Build history of the part. All positions in model axes, mm. A direction names the side the tool comes from. Give positions to 0.01 mm unless a question says otherwise; leave off trailing zeros. Order: outer loops, then holes, each group sorted by start corner. A loop starts at its lowest first (then second) coordinate and runs counter-clockwise, first axis right, second up. Notation, with made-up numbers: (87, 29) - (101, 29) arc R9 cw to (101, 42) - close; hole circle Ø2 at (-27.75, -15.75). An arc over 180 degrees is marked (long way). Use a Markdown table: item, result. Add a question column.
(1) Slice it at A-A (z = -39). Write the cut outline in (x, y).
(2) Flat gauge pins, fed straight in: pin 1 (6 mm diameter, centred on x = 223, y = 4.5, fed in from +Z); pin 2 (11.5 mm diameter, centred on x = 39.03, z = -19.51, fed in from -Y); pin 3 (6 mm diameter, centred on x = 59, y = 79, fed in from +Z). Where does each tip first touch, or does it go through?
(3) Which spindle directions (+Z, -Z, +X, -X, +Y, -Y) get a long thin tool onto all of the face, cutting with end or side? Do faces 4 (the face through (155, 7.62, -69)), 5 (the face through (138.825, 97.843, -52.046)), 6 (the face through (221.732, 95.161, -148.505)). Say none if no direction does.
(4) Slice it at D-D (y = 43). Write the cut outline in (x, z).
(5) Wall check: line 1 (Y direction, x = 155.5, z = -60.5); line 2 (X direction, y = 6.5, z = -4); line 3 (X direction, y = 96.5, z = 0). Give the ranges that are in metal, low to high.
(6) Slice it at B-B (x = 162). Write the cut outline in (y, z), then the cut area to 3 significant figures.
(7) Mould opens along X. For faces 1 (the face through (89, 95, -89)), 2 (the face through (143, 93.98, -52)), 3 (the face through (194.36, 6.26, -166.13)) say: +X half, -X half, draft (parallel to the pull), parting line (faces both ways), or undercut.
(8) Slice it at C-C (z = -3). Write the cut outline in (x, y).
from build123d import *

# Parameters (mm, degrees)
BOSS_EXTRUDE1_DEPTH = 101.6
SKETCH2_W           = 267.926874414
SKETCH2_H           = 76.2
CUT_EXTRUDE1_DEPTH  = 71.12
SKETCH3_R           = 6.35
CUT_EXTRUDE3_DEPTH  = 313.194791695
CUT_EXTRUDE4_DEPTH  = 7.62
CUT_EXTRUDE5_DEPTH  = 7.62


with BuildPart() as part:
    # Sketch1 → Boss-Extrude1 (new body)
    with BuildSketch(Plane(origin=(0, 0, 0), x_dir=(1, 0, 0), z_dir=(0, 1, 0))):
        Polygon((0, 0), (179.605122421, 179.605122421), (209.535625582, 152.272255569), (234.275538547, 144.630280974), (62.844388347, -43.093188015), align=None)
    extrude(amount=BOSS_EXTRUDE1_DEPTH)

    # Sketch2 → Cut-Extrude1 (cut)
    with BuildSketch(Plane(origin=(0, 0, 0), x_dir=(-0.7071067811865464, 0, 0.7071067811865487), z_dir=(-0.7071067811865487, 0, -0.7071067811865464))):
        with Locations((-133.963437207, 50.8)):
            Rectangle(SKETCH2_W, SKETCH2_H)
    extrude(amount=-CUT_EXTRUDE1_DEPTH, mode=Mode.SUBTRACT)

    # Sketch3 → Cut-Extrude3 (cut, through all)
    with BuildSketch(Plane(origin=(0, 101.6, 0), x_dir=(1, 0, 0), z_dir=(0, 1, 0))):
        with Locations(Location((21.07252481, 1.552947287, 0), (0, 0, 270))):
            Circle(SKETCH3_R)
        with Locations(Location((39.033037052, 19.513459529, 0), (0, 0, 270))):
            Circle(SKETCH3_R)
        with Locations(Location((56.993549294, 37.473971772, 0), (0, 0, 270))):
            Circle(SKETCH3_R)
        with Locations(Location((74.954061536, 55.434484014, 0), (0, 0, 270))):
            Circle(SKETCH3_R)
        with Locations(Location((92.914573778, 73.394996256, 0), (0, 0, 270))):
            Circle(SKETCH3_R)
        with Locations(Location((110.87508602, 91.355508498, 0), (0, 0, 270))):
            Circle(SKETCH3_R)
        with Locations(Location((128.835598263, 109.31602074, 0), (0, 0, 270))):
            Circle(SKETCH3_R)
        with Locations(Location((146.796110505, 127.276532982, 0), (0, 0, 270))):
            Circle(SKETCH3_R)
        with Locations(Location((164.756622747, 145.237045224, 0), (0, 0, 270))):
            Circle(SKETCH3_R)
    extrude(amount=-CUT_EXTRUDE3_DEPTH, mode=Mode.SUBTRACT)

    # Sketch4 → Cut-Extrude4 (cut)
    with BuildSketch(Plane(origin=(0, 101.6, 0), x_dir=(1, 0, 0), z_dir=(0, 1, 0))):
        Polygon((57.221000047, -36.701269589), (222.746181499, 143.313374464), (227.72700376, 141.940671831), (60.924166757, -39.463469017), align=None)
    extrude(amount=-CUT_EXTRUDE4_DEPTH, mode=Mode.SUBTRACT)

    # Sketch5 → Cut-Extrude5 (cut)
    with BuildSketch(Plane(origin=(0, 0, 0), x_dir=(-1, 0, 0), z_dir=(0, -1, 0))):
        Polygon((-218.913299563, 144.742548401), (-62.856752097, -25.376237408), (-58.071451081, -30.592741372), (-62.856752097, -34.982483231), (-227.725480711, 144.742548401), align=None)
    extrude(amount=-CUT_EXTRUDE5_DEPTH, mode=Mode.SUBTRACT)


solid = part.part
Solution:
| question | item | result |
|---|---|---|
| 1 | outline | (39, 0) - (50.83, 0) - (50.83, 12.7) - (39, 12.7) - close; (39, 88.9) - (50.83, 88.9) - (50.83, 101.6) - (39, 101.6) - close; (63.16, 0) - (121.91, 0) - (121.91, 7.62) - (130.72, 7.62) - (130.72, 0) - (137.81, 0) - (137.81, 12.7) - (63.16, 12.7) - close; (63.16, 88.9) - (137.81, 88.9) - (137.81, 101.6) - (133.07, 101.6) - (133.07, 93.98) - (126.83, 93.98) - (126.83, 101.6) - (63.16, 101.6) - close |
| 2 | pin 1 | z = -129 |
| 2 | pin 2 | through |
| 2 | pin 3 | z = 42.51 |
| 3 | face 4 | -Y |
| 3 | face 5 | +Y |
| 3 | face 6 | -Z, +X, +Y, -Y |
| 4 | outline | (59.67, 40.91) - (119.23, -18.65) - (62.84, 43.09) - close |
| 5 | line 1 | 0 to 12.7, 88.9 to 101.6 |
| 5 | line 2 | 4 to 15.21, 26.93 to 89.8, 98.62 to 105.85 |
| 5 | line 3 | 0 to 14.92, 27.23 to 90.97, 97.21 to 102.2 |
| 6 | outline | (0, -162) - (12.7, -162) - (12.7, -150.96) - (0, -150.96) - close; (0, -139.52) - (12.7, -139.52) - (12.7, -65.49) - (0, -65.49) - (0, -73.09) - (7.62, -73.09) - (7.62, -82.7) - (0, -82.7) - close; (88.9, -162) - (101.6, -162) - (101.6, -150.96) - (88.9, -150.96) - close; (88.9, -139.52) - (101.6, -139.52) - (101.6, -77.25) - (93.98, -77.25) - (93.98, -70.46) - (101.6, -70.46) - (101.6, -65.49) - (88.9, -65.49) - close |
| 6 | area | 2,040 mm2 |
| 7 | face 1 | -X half |
| 7 | face 2 | undercut |
| 7 | face 3 | +X half |
| 8 | outline | (3, 0) - (14.89, 0) - (14.89, 12.7) - (3, 12.7) - close; (3, 88.9) - (14.89, 88.9) - (14.89, 101.6) - (3, 101.6) - close; (27.26, 0) - (88.89, 0) - (88.89, 7.62) - (97.7, 7.62) - (97.7, 0) - (104.94, 0) - (104.94, 101.6) - (99.97, 101.6) - (99.97, 93.98) - (93.73, 93.98) - (93.73, 101.6) - (27.26, 101.6) - (27.26, 88.9) - (103.58, 88.9) - (103.58, 12.7) - (27.26, 12.7) - close |
